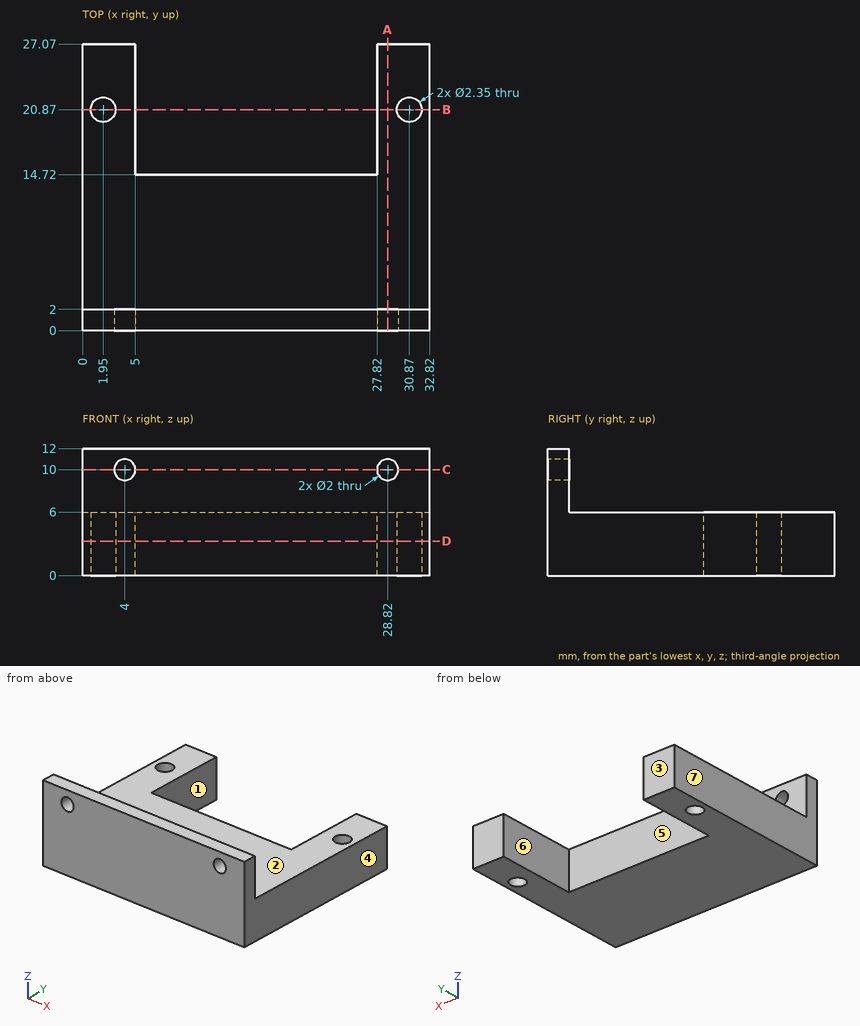
Could you check a few things on this drawing? It's one solid part, dimensions in mm from its lowest x, y, z. A direction names the side the tool comes from. Give positions to 0.01 mm unless a question says otherwise; leave off trailing zeros. Write each loop counter-clockwise with the first axis right and the second up, starting at its lowest first coordinate (ties: lowest second). Pieces come first, ordered by that corner, then holes. Notation, with made-up numbers: M -1,-21.5 L 14,-21.5 A19 cw 14,-4.5 Z; hole C 31.25,41 d10. An arc over 180 degrees is marked long. Put each result on its own line as item: value. Start each with the question number.
Item 1: On a 3-axis mill with a long thin cutter (end or side, diameter ignored), from which of +Z, -Z, +X, -X, +Y, -Y can I reach the whole of each face in a straight line? I mean the marked faces 1, 2 and 3. Say none if no direction works.
Item 2: If we section it at B-B, the plane y = 20.87: Write out the boundary of the cut face in (x, z) (3 decimals), then the cut area to 3 significant figures.
Item 3: If we section it at C-C, the plane z = 10: Write out the boundary of the cut face in (x, y), then the cut area to 3 significant figures.
Item 4: Thinking about a two-plate mould opening in X: for the marked faces 4, 5, 6 and 7, which applies, +X half, -X half, draft (parallel to the pull), parting line (faces both ways), or undercut?
Item 5: Will these pins go through, and if not, where does the flat tip stop? pin 1 (6.5 mm diameter, centred on x = 16.5, z = 8, fed in from +Y); pin 2 (1.8 mm diameter, centred on x = 4, z = 10, fed in from +Y); pin 3 (3 mm diameter, centred on x = 30.87, y = 20.87, fed in from +Z); pin 4 (2 mm diameter, centred on y = 15, z = 5, fed in from -X).
Item 6: If we section it at D-D, the plane z = 3.25: Write out the boundary of the cut face in (x, y) (3 decimals), then the cut area to 3 significant figures.
Item 7: I need wall thicknesses on L1, parallel to X at y = 1.5, z = 10; L2, parallel to Y at x = 1.95, z = 3.45 (3 decimals); L3, parallel to Z at x = 4, y = 0.4. Which ranges of each line are inside material? Lowest first, please. Write a range as from..to.
Item 8: If we section it at A-A, the plane x = 28.82: Write out the boundary of the cut face in (y, z).
Values:
1. face 1: +Z, -Z, +Y
1. face 2: +Z, +X, -X, +Y
1. face 3: +Z, -Z, +X, -X, +Y
2. outline: M 0,0 L 0.775,0 L 0.775,6 L 0,6 Z; M 3.125,0 L 5,0 L 5,6 L 3.125,6 Z; M 27.82,0 L 29.695,0 L 29.695,6 L 27.82,6 Z; M 32.045,0 L 32.82,0 L 32.82,6 L 32.045,6 Z
2. area: 31.8 mm²
3. outline: M 0,0 L 3,0 L 3,2 L 0,2 Z; M 5,0 L 27.82,0 L 27.82,2 L 5,2 Z; M 29.82,0 L 32.82,0 L 32.82,2 L 29.82,2 Z
3. area: 57.6 mm²
4. face 4: +X half
4. face 5: undercut
4. face 6: undercut
4. face 7: -X half
5. pin 1: y = 14.72
5. pin 2: through
5. pin 3: z = 6
5. pin 4: x = 0
6. outline: M 0,0 L 32.82,0 L 32.82,27.07 L 27.82,27.07 L 27.82,14.72 L 5,14.72 L 5,27.07 L 0,27.07 Z; hole C 1.95,20.87 d2.35; hole C 30.87,20.87 d2.35
6. area: 598 mm²
7. L1: 0..3, 5..27.82, 29.82..32.82
7. L2: 0..19.695, 22.045..27.07
7. L3: 0..9, 11..12
8. outline: M 0,0 L 27.07,0 L 27.07,6 L 2,6 L 2,9 L 0,9 Z; M 0,11 L 2,11 L 2,12 L 0,12 Z
